Print and shaded views of the part. All mm, measured from the part's lowest x, y and z. A direction names the side the tool comes from. Round coordinates to 2 decimals unless told otherwise and drop trailing zeros. Write each loop counter-clockwise with the first axis right and the second up, starting at its lowest first coordinate (ties: lowest second). Pieces come first, ordered by that corner, then holes. Notation, with made-up numbers: M 81,18 L 99,18 A25 ccw 99,33 Z; hole C 27,-15.75 d2. An arc over 180 degrees is marked long. Write item = value, one per line. Start each with the question number.
Q1. Band-saw the part on C-C on z = 1.75. Write the cut outline in (x, y), plus the area to 3 significant figures.
Q2. Probe L1, parallel to Y at x = 59.5, z = 6.5; L2, parallel to X at y = 29.5, z = 16; L3, parallel to Y at x = 24, z = 8. List the from-to ranges inside material, lowest first.
Q3. Band-saw the part on A-A on x = 40. Write the cut outline in (y, z), plus the area to 3 significant figures.
Q4. Band-saw the part on D-D on y = 33. Write the cut outline in (x, z).
Q5. Drop flat-ended pins along their axis: P1, Ø5.5, axis at y = 27.5, z = 10, coming from the +X side; P2, Ø7, axis at x = 20.5, y = 4.5, coming from the +Z side; P3, Ø2, axis at x = 1, z = 2.5, coming from the +Y side. Give the stop position or say it passes through.
Q6. Pull direction Y, two halves, no side cores. Call the marked faces 3, 4, 5 and 6: released by +Y, released by -Y, zero draft, split by the parting line, or undercut.
Q7. Band-saw the part on B-B on y = 4.5. Write the cut outline in (x, z).
Q8. Tool access for the marked faces 1 and 2: list every direction of +Z, -Z, +X, -X, +Y, -Y with a clear straight run to the whole face (end or side of a thin tool).
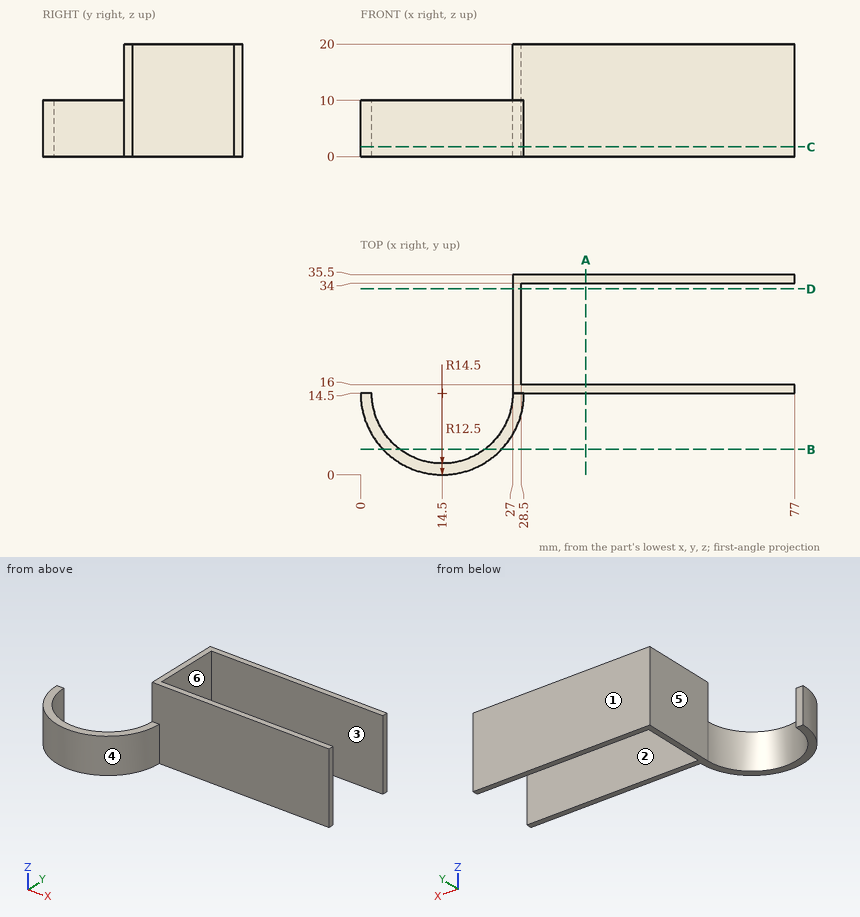
Conclusion:
q1.outline = M 0,14.5 A14.5 ccw 29,14.5 L 77,14.5 L 77,16 L 28.5,16 L 28.5,34 L 77,34 L 77,35.5 L 27,35.5 L 27,14.5 A12.5 cw 2,14.5 Z
q1.area = 262 mm^2
q2.L1 = 14.5 to 16, 34 to 35.5
q2.L2 = 27 to 28.5
q2.L3 = 3.55 to 6.38
q3.outline = M 14.5,0 L 16,0 L 16,20 L 14.5,20 Z; M 34,0 L 35.5,0 L 35.5,20 L 34,20 Z
q3.area = 60.0 mm^2
q4.outline = M 27,0 L 28.5,0 L 28.5,20 L 27,20 Z
q5.P1 = 28.5
q5.P2 = 10
q5.P3 = 14.5
q6.face_3 = undercut
q6.face_4 = released by -Y
q6.face_5 = zero draft
q6.face_6 = undercut
q7.outline = M 4,0 L 7,0 L 7,10 L 4,10 Z; M 22,0 L 25,0 L 25,10 L 22,10 Z
q8.face_1 = +Z, -Z, +X, -X, +Y
q8.face_2 = +Z, -Z, +X
